```python
from build123d import *

# Parameters (mm, degrees)
BOSS_EXTRUDE1_DEPTH = 4.5
SKETCH2_W           = 9
SKETCH2_H           = 10
BOSS_EXTRUDE2_DEPTH = 4.5
BOSS_EXTRUDE3_DEPTH = 4.5
CUT_EXTRUDE1_DEPTH  = 84.792899461
SKETCH5_W           = 10
SKETCH5_H           = 9
BOSS_EXTRUDE4_DEPTH = 4.5
CUT_EXTRUDE2_DEPTH  = 84.792899461


with BuildPart() as part:
    # Sketch1 → Boss-Extrude1 (new body)
    with BuildSketch(Plane(origin=(0, 0, 0), x_dir=(0, 0, -1), z_dir=(1, 0, 0))):
        Polygon((0, 0), (0, -35), (-76, 0), align=None)
    extrude(amount=BOSS_EXTRUDE1_DEPTH)

    # Sketch2 → Boss-Extrude2 (add, through all)
    with BuildSketch(Plane(origin=(4.5, 0, 0), x_dir=(0, 0, -1), z_dir=(1, 0, 0))):
        with Locations((0, -7.5)):
            Rectangle(SKETCH2_W, SKETCH2_H)
    extrude(amount=-BOSS_EXTRUDE2_DEPTH)

    # Sketch3 → Boss-Extrude3 (add, through all)
    with BuildSketch(Plane(origin=(4.5, 0, 0), x_dir=(0, 0, -1), z_dir=(1, 0, 0))):
        Polygon((0, -35), (-15, -35), (-76, 0), (0, -25), align=None)
    extrude(amount=-BOSS_EXTRUDE3_DEPTH)

    # Sketch4 → Cut-Extrude1 (cut, through all)
    with BuildSketch(Plane(origin=(4.5, 0, 0), x_dir=(0, 0, -1), z_dir=(1, 0, 0))):
        with BuildLine():
            Line((0, -31.25), (0, -27.75))
            Line((0, -27.75), (-3.8, -27.75))
            Line((-3.8, -27.75), (-3.8, -26.75))
            ThreePointArc((-3.8, -26.75), (-3.873223305, -26.573223305), (-4.05, -26.5))
            Line((-4.05, -26.5), (-7.75, -26.5))
            ThreePointArc((-7.75, -26.5), (-7.926776695, -26.573223305), (-8, -26.75))
            Line((-8, -26.75), (-8, -27.75))
            Line((-8, -27.75), (-10.5, -27.75))
            Line((-10.5, -27.75), (-10.5, -31.25))
            Line((-10.5, -31.25), (-8, -31.25))
            Line((-8, -31.25), (-8, -32.25))
            ThreePointArc((-8, -32.25), (-7.926776695, -32.426776695), (-7.75, -32.5))
            Line((-7.75, -32.5), (-4.05, -32.5))
            ThreePointArc((-4.05, -32.5), (-3.873223305, -32.426776695), (-3.8, -32.25))
            Line((-3.8, -32.25), (-3.8, -31.25))
            Line((-3.8, -31.25), (0, -31.25))
        make_face()
    extrude(amount=-CUT_EXTRUDE1_DEPTH, mode=Mode.SUBTRACT)

    # Sketch5 → Boss-Extrude4 (add, through all)
    with BuildSketch(Plane(origin=(4.5, 0, 0), x_dir=(0, 0, -1), z_dir=(1, 0, 0))):
        with Locations((-20, 0)):
            Rectangle(SKETCH5_W, SKETCH5_H)
        with Locations((-45, 0)):
            Rectangle(SKETCH5_W, SKETCH5_H)
    extrude(amount=-BOSS_EXTRUDE4_DEPTH)

    # Sketch6 → Cut-Extrude2 (cut, through all)
    with BuildSketch(Plane(origin=(4.5, 0, 0), x_dir=(0, 0, -1), z_dir=(1, 0, 0))):
        with BuildLine():
            Line((-30.75, 0), (-34.25, 0))
            Line((-34.25, 0), (-34.25, -3.8))
            Line((-34.25, -3.8), (-35.25, -3.8))
            ThreePointArc((-35.25, -3.8), (-35.426776695, -3.873223305), (-35.5, -4.05))
            Line((-35.5, -4.05), (-35.5, -7.75))
            ThreePointArc((-35.5, -7.75), (-35.426776695, -7.926776695), (-35.25, -8))
            Line((-35.25, -8), (-34.25, -8))
            Line((-34.25, -8), (-34.25, -10.5))
            Line((-34.25, -10.5), (-30.75, -10.5))
            Line((-30.75, -10.5), (-30.75, -8))
            Line((-30.75, -8), (-29.75, -8))
            ThreePointArc((-29.75, -8), (-29.573223305, -7.926776695), (-29.5, -7.75))
            Line((-29.5, -7.75), (-29.5, -4.05))
            ThreePointArc((-29.5, -4.05), (-29.573223305, -3.873223305), (-29.75, -3.8))
            Line((-29.75, -3.8), (-30.75, -3.8))
            Line((-30.75, -3.8), (-30.75, 0))
        make_face()
    extrude(amount=-CUT_EXTRUDE2_DEPTH, mode=Mode.SUBTRACT)


solid = part.part
```
Design review of the part built by this model. Coordinates are the model's own, in mm. A direction names the side the tool comes from. Coordinates: 2 decimals unless noted, no trailing zeros. Write each loop counter-clockwise with the first axis right and the second up, starting at its lowest first coordinate (ties: lowest second). Pieces come first, ordered by that corner, then holes. Notation, with made-up numbers: M 33,71 L 79,71 A20 cw 79,86 Z; hole C 18,-4.75 d1. An arc over 180 degrees is marked long. Answer as a JSON object with one key per item and string values.
Item 1: Draft analysis for pull direction Z (two halves, no side actions). For faces 1 (the flat face through (2, 0, 8)), 2 (the flat face through (2, -32.5, 6)), 3 (the flat face through (2, -29, 10.5)), state which applies: pulls with the +Z half, pulls with the -Z half, needs draft (parallel to the pull), parting line crosses it, or undercut.
Outcome:
{"face 1": "needs draft", "face 2": "undercut", "face 3": "pulls with the -Z half"}
Item 2: Add section B-B, the plane z = 64.5. Give the boundary of the cut face in (x, y), and give its area (3 significant figures).
Outcome:
{"outline": "M 0,-6.6 L 4.5,-6.6 L 4.5,0 L 0,0 Z", "area": "29.7 mm²"}
Item 3: Wall thickness on probe 1 along Y at (x, z) = (1.65, 4.5); probe 2 along Z at (x, y) = (3.25, 2.5); probe 3 along Y at (x, z) = (1.9, 2.5): over which ranges is each line inside the solid? List them lowest first.
Outcome:
{"probe 1": "-35 to -32.5, -26.5 to 0", "probe 2": "15 to 25, 40 to 50", "probe 3": "-35 to -31.25, -27.75 to 0"}
Item 4: Machinability: for faces 4 (the flat face through (2, -6, 29.5)), 5 (the flat face through (2, -31.25, 9)), 6 (the flat face through (2, -12.5, -2)), 7 (the flat face through (2, -9, 30.75)), which of the approach directions +Z, -Z, +X, -X, +Y, -Y give a long, thin tool a straight path to every point of the face, cutting with its end or side? Answer none if there is none.
Outcome:
{"face 4": "+X, -X", "face 5": "-Z, +X, -X", "face 6": "-Z, +X, -X, -Y", "face 7": "+X, -X, +Y"}
Item 5: Insertion check: pin 1 Ø1 at (x, y) = (3.5, -16.5) entering from -Z; pin 2 Ø1.1 at (x, z) = (2, 30) entering from -Y; pin 3 Ø12 at (y, z) = (-26.5, 51) entering from -X; pin 4 Ø1.3 at (x, z) = (3.5, -2.5) entering from -Y. Each pin has a flat end and moves straight along its axis. Give the tip position at first contact, or say it passes through.
Outcome:
{"pin 1": "z = 0", "pin 2": "y = -26.71", "pin 3": "through", "pin 4": "y = -12.5"}
Item 6: Add section C-C, the plane y = -25. Give the boundary of the cut face in (x, z), and give its area (3 significant figures).
Outcome:
{"outline": "M 0,0 L 4.5,0 L 4.5,32.43 L 0,32.43 Z", "area": "146 mm²"}
Item 7: Add section A-A, the plane y = -9. Give the boundary of the cut face in (x, z).
Outcome:
{"outline": "M 0,-4.5 L 4.5,-4.5 L 4.5,30.75 L 0,30.75 Z; M 0,34.25 L 4.5,34.25 L 4.5,60.31 L 0,60.31 Z"}
